```python
from build123d import *

# Parameters (mm, degrees)
F1_DEPTH    = 80
F2_T1_DEPTH = 140
F2_T3_DEPTH = 85
F2_T6_ANGLE = 90
F2_T8_ANGLE = 90
F3_W        = 30
F3_H        = 80
F4_DEPTH    = 25


# Not quite as in the source:
# - a fillet or chamfer that OpenCascade refuses, or shapes differently, is made with other operations: its cross-section is extruded or revolved along the edge and cut away or added


with BuildPart() as f1:
    # F0 (on Front) → F1 (new body)
    with BuildSketch(Plane.XZ):
        with BuildLine():
            Line((85, 129.9038105677), (75, 129.9038105677))
            Line((75, 129.9038105677), (0, 0))
            Line((0, 0), (16.9389196682, 0))
            Line((16.9389196682, 0), (16.9389196682, 4.9038105677))
            Line((16.9389196682, 4.9038105677), (34.5854811567, 4.9038105677))
            Line((34.5854811567, 4.9038105677), (34.5854811567, 6.5063509461))
            ThreePointArc((34.5854811567, 6.5063509461), (36.2891898423, 19.4473032012), (41.2842109675, 31.5063509461))
            Line((41.2842109675, 31.5063509461), (86.5319459163, 109.8777268049))
            ThreePointArc((86.5319459163, 109.8777268049), (117.3568969946, 96.1773012088), (130, 64.9038105677))
            ThreePointArc((130, 64.9038105677), (127.4711560413, 41.3606586971), (120, 18.8916382651))
            Line((120, 18.8916382651), (120, 4.9038105677))
            Line((120, 4.9038105677), (135, 4.9038105677))
            Line((135, 4.9038105677), (135, -0.0961894323))
            Line((135, -0.0961894323), (150, -0.0961894323))
            Line((150, -0.0961894323), (150, 64.9038105677))
            ThreePointArc((150, 64.9038105677), (130.9619407771, 110.8657513448), (85, 129.9038105677))
        make_face()
    extrude(amount=F1_DEPTH)

    # F2: fillet of radius 30 on 2 edges, made by hand

    # F2_s2 → F2_t1 (cut)
    with BuildSketch(Plane.XY.offset(-75.0961894323)):
        with BuildLine():
            ThreePointArc((150, -50), (141.2132034356, -71.2132034356), (120, -80))
            Line((120, -80), (150, -80))
            Line((150, -80), (150, -50))
        make_face()
        with BuildLine():
            ThreePointArc((150, -30), (141.2132034356, -8.7867965644), (120, 0))
            Line((120, 0), (150, 0))
            Line((150, 0), (150, -30))
        make_face()
    extrude(amount=F2_T1_DEPTH, mode=Mode.SUBTRACT)

    # F2_s4 → F2_t3 (cut)
    with BuildSketch(Plane.YZ):
        with BuildLine():
            ThreePointArc((-50, 129.9038105677), (-71.2132034356, 121.1170140033), (-80, 99.9038105677))
            Line((-80, 99.9038105677), (-80, 129.9038105677))
            Line((-80, 129.9038105677), (-50, 129.9038105677))
        make_face()
        with BuildLine():
            ThreePointArc((-30, 129.9038105677), (-8.7867965644, 121.1170140033), (0, 99.9038105677))
            Line((0, 99.9038105677), (0, 129.9038105677))
            Line((0, 129.9038105677), (-30, 129.9038105677))
        make_face()
    extrude(amount=F2_T3_DEPTH, mode=Mode.SUBTRACT)

    # F2_s5 → F2_t6 (revolve, cut)
    with BuildSketch(Plane.XY.offset(64.9038105677)):
        with BuildLine():
            ThreePointArc((150, -30), (141.2132034356, -8.7867965644), (120, 0))
            Line((120, 0), (150, 0))
            Line((150, 0), (150, -30))
        make_face()
    revolve(axis=Axis((85, 0, 64.9038105677), (0, -1, 0)), revolution_arc=F2_T6_ANGLE, mode=Mode.SUBTRACT)

    # F2_s7 → F2_t8 (revolve, cut)
    with BuildSketch(Plane.XY.offset(64.9038105677)):
        with BuildLine():
            ThreePointArc((150, -50), (141.2132034356, -71.2132034356), (120, -80))
            Line((120, -80), (150, -80))
            Line((150, -80), (150, -50))
        make_face()
    revolve(axis=Axis((85, -80, 64.9038105677), (0, -1, 0)), revolution_arc=F2_T8_ANGLE, mode=Mode.SUBTRACT)


with BuildPart() as f4:
    # F3 (on Top) → F4 (new body)
    with BuildSketch(Plane.XY):
        with Locations((140.605225563, -40)):
            Rectangle(F3_W, F3_H)
    extrude(amount=F4_DEPTH)

    # F5: cut F1
    add(f1.part, mode=Mode.SUBTRACT)


solid = f4.part
```
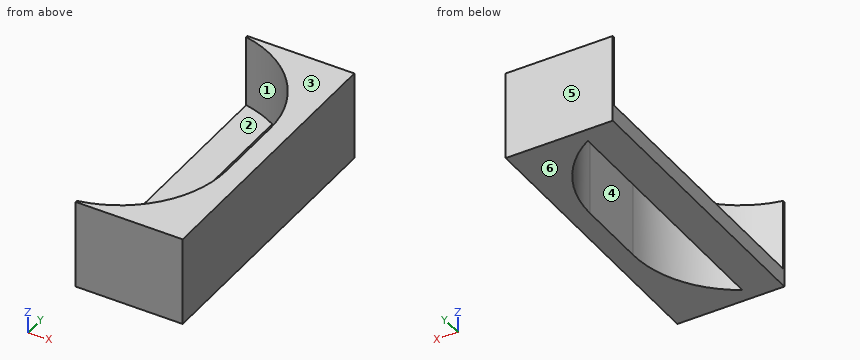
Model file for the job. Use its own axes, mm. Face numbers are marked on the shaded views. A direction names the side the tool comes from. Coordinates: 2 decimals unless noted, no trailing zeros. Loops run counter-clockwise (first coordinate to the right, second up) from the corner with the lowest first, then second, coordinate; pieces in that order, holes last. Notation, with made-up numbers: (76.25, -11.75) - (133.25, -11.75) arc R36 ccw to (133.25, 25.25) - close; hole circle Ø3 at (22.5, 3.5). An arc over 180 degrees is marked (long way). Write item = value, one per line. Start each with the question number.
Item 1: Saw through at A-A, the plane y = -36.5. List the corners of the cut face in (x, z).
Item 2: Saw through at B-B, the plane x = 145. List the corners of the cut face in (y, z).
Item 3: Saw through at C-C, the plane z = 3.5. List the corners of the cut face in (x, y).
Item 4: Wall check: probe 1 along X at (y, z) = (-51, 2.5); probe 2 along Y at (x, z) = (146.5, 20.75); probe 3 along X at (y, z) = (-61, 4). Give the ranges that are in metal, low to high. Write a range as [from, to].
Item 5: Saw through at D-D, the plane z = 20.5. List the corners of the cut face in (x, y), then the cut area to 3 significant figures.
Item 6: Pull direction Y, two halves, no side cores. Call the marked faces 4, 5 and 6: +Y half, -Y half, draft (parallel to the pull), parting line (faces both ways), or undercut.
Item 7: Drop flat-ended pins along their axis: pin 1 Ø3 at (x, y) = (130.5, -51.5) entering from +Z; pin 2 Ø1.5 at (y, z) = (-70, 11.5) entering from -X. Give the stop position or say it passes through.
Item 8: 3-axis set-ups, long thin cutter, end or side, ignore diameter. For the marked faces 1, 2 and 3: which of +Z, -Z, +X, -X, +Y, -Y reach the whole face in a straight line?
Answers:
q1.outline = (125.61, 0) - (135, 0) - (135, 4.9) - (125.61, 4.9) - close; (150, 0) - (155.61, 0) - (155.61, 25) - (150, 25) - close
q2.outline = (-80, 0) - (-66.58, 0) - (-66.58, 25) - (-80, 25) - close; (-13.42, 0) - (0, 0) - (0, 25) - (-13.42, 25) - close
q3.outline = (125.61, -80) - (155.61, -80) - (155.61, 0) - (125.61, 0) - close; hole (135, -75.98) arc R30 ccw to (150, -50) - (150, -30) arc R30 ccw to (135, -4.02) - close
q4.probe_1 = [125.61, 135], [149.98, 155.61]
q4.probe_2 = [-80, -64.06], [-15.94, 0]
q4.probe_3 = [125.61, 135], [147.91, 155.61]
q5.outline = (125.61, -80) - (155.61, -80) - (155.61, 0) - (125.61, 0) - (125.61, -0.53) arc R30 cw to (150, -30) - (150, -50) arc R30 cw to (125.61, -79.47) - close
q5.area = 833 mm2
q6.face_4 = undercut
q6.face_5 = +Y half
q6.face_6 = draft
q7.pin_1 = 4.9
q7.pin_2 = 141.67
q8.face_1 = +Z
q8.face_2 = +Z, -X
q8.face_3 = +Z, +X, -X, +Y, -Y
